Design review of the part shown in the three views and the two pictorial views. Dimensions are in mm from the part's minimum x, y and z. A direction names the side the tool comes from. Coordinates: 2 decimals unless noted, no trailing zeros. Order: outer loops, then holes, each group sorted by start corner. A loop starts at its lowest first (then second) coordinate and runs counter-clockwise, first axis right, second up. Notation, with made-up numbers: (17.25, 83) -> (27.25, 83) arc R22 cw to (27.25, 90) -> close; hole circle Ø7 at (-0.5, 51). An arc over 180 degrees is marked (long way). Answer as a JSON object with one key per item and string values. Group by question number.
1) Add section B-B, the plane x = 26. Write out the cut boundary in (y, z), then the cut area to 4 significant figures.
2) Machinability: for the marked faces 4, 5 and 6, which of the approach directions +Z, -Z, +X, -X, +Y, -Y give a long, thin tool a straight path to every point of the face, cutting with its end or side? Answer none if there is none.
3) Draft analysis for pull direction Y (two halves, no side actions). For the marked faces 1, 2 and 3, state which applies: +Y half, -Y half, draft (parallel to the pull), parting line (faces both ways), or undercut.
4) Add section C-C, the plane y = 23.5. Write out the cut boundary in (x, z), then the cut area to 3 significant figures.
5) Add section A-A, the plane z = 1.25. Write out the cut boundary in (x, y).
6) Add section D-D, the plane x = 47. Write out the cut boundary in (y, z), then the cut area to 3 significant figures.
7) For pin 1 (17.5 mm diameter, centred on x = 26, y = 20, fed in from -Z); pin 2 (3 mm diameter, centred on x = 47, z = 5.5, fed in from +Y); pin 3 (5 mm diameter, centred on y = 20, z = 5.5, fed in from +X); pin 4 (5 mm diameter, centred on x = 18, z = 1.5, fed in from +Y) (3 decimals), all flat-tipped, find the tip position at first contact; note any pin that passes through.
8) Wall thickness on L1, parallel to Y at x = 26, z = 3.25; L2, parallel to X at y = 20, z = 8.6; L3, parallel to Y at x = 26, z = 9.3: over which ranges is each line inside the solid? List them lowest first.
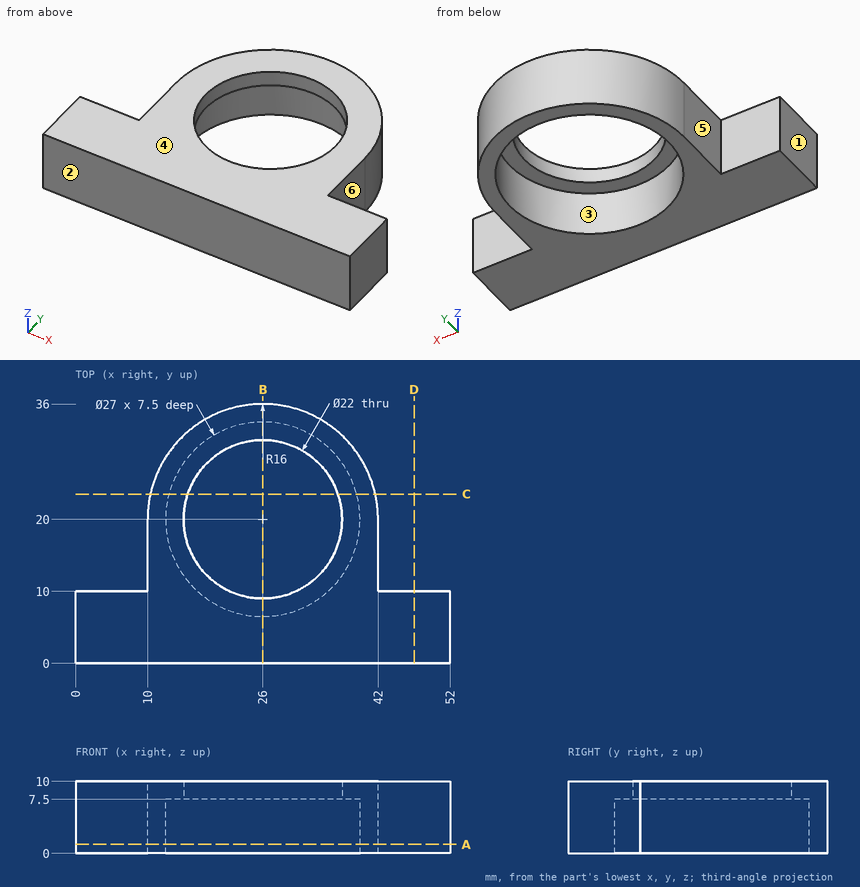
Output values:
{
 "1": {"outline": "(0, 0) -> (6.5, 0) -> (6.5, 7.5) -> (9, 7.5) -> (9, 10) -> (0, 10) -> close; (31, 7.5) -> (33.5, 7.5) -> (33.5, 0) -> (36, 0) -> (36, 10) -> (31, 10) -> close", "area": "102.5 mm²"},
 "2": {"face 4": "+Z, +X, -X, +Y, -Y", "face 5": "+Z, -Z, -X, +Y", "face 6": "+Z, -Z, +X, +Y"},
 "3": {"face 1": "draft", "face 2": "-Y half", "face 3": "undercut"},
 "4": {"outline": "(10.39, 0) -> (12.96, 0) -> (12.96, 7.5) -> (15.57, 7.5) -> (15.57, 10) -> (10.39, 10) -> close; (36.43, 7.5) -> (39.04, 7.5) -> (39.04, 0) -> (41.61, 0) -> (41.61, 10) -> (36.43, 10) -> close", "area": "64.5 mm²"},
 "5": {"outline": "(0, 0) -> (52, 0) -> (52, 10) -> (42, 10) -> (42, 20) arc R16 ccw to (10, 20) -> (10, 10) -> (0, 10) -> close; hole circle Ø27 at (26, 20)"},
 "6": {"outline": "(0, 0) -> (10, 0) -> (10, 10) -> (0, 10) -> close", "area": "100 mm²"},
 "7": {"pin 1": "passes through", "pin 2": "stops at y = 10", "pin 3": "stops at x = 42", "pin 4": "stops at y = 35.025"},
 "8": {"L1": "y = 0 to 6.5, 33.5 to 36", "L2": "x = 10 to 15, 37 to 42", "L3": "y = 0 to 9, 31 to 36"}
}
